For this review, take the finished solid that the model builds, in its own axes (mm). A direction names the side the tool comes from. Round coordinates to 2 decimals unless told otherwise and drop trailing zeros. Write each loop counter-clockwise with the first axis right and the second up, starting at its lowest first coordinate (ties: lowest second). Pieces come first, ordered by that corner, then holes. Notation, with made-up numbers: (-14, 68) -> (25, 68) arc R17 ccw to (25, 93) -> close; hole circle Ø10 at (6.5, -16.5). An arc over 180 degrees is marked (long way). Answer in a Markdown table with one row per item.
from build123d import *

# Parameters (mm, degrees)
SKETCH1_W                             = 69.85
SKETCH1_H                             = 25.4
EXTRUDE1_DEPTH                        = 1.5748
F_1_8_0_125_DIAMETER_HOLE1_AT_2_COUNT = 2
F_1_8_0_125_DIAMETER_HOLE1_AT_2_PITCH = 57.13222
SKETCH4_R                             = 0.635
BOSS_EXTRUDE1_DEPTH                   = 177.8
SKETCH5_W                             = 8.128
SKETCH5_H                             = 8.7376
USB_CONNECTOR_DEPTH                   = 4.1402
SKETCH6_W                             = 10.40639215
SKETCH6_H                             = 6.781860105
CHARGER_DEPTH                         = 20.828
SKETCH7_W                             = 6.585703948
SKETCH7_H                             = 3.257259008
BOSS_EXTRUDE2_DEPTH                   = 10.16
SKETCH8_W                             = 6.5278
SKETCH8_H                             = 15.6718
BOSS_EXTRUDE3_DEPTH                   = 9.8298


with BuildPart() as part:
    # Sketch1 → Extrude1 (new body)
    with BuildSketch(Plane.XY):
        Rectangle(SKETCH1_W, SKETCH1_H)
    extrude(amount=EXTRUDE1_DEPTH)

    # Sketch3 → 1/8 (0.125) Diameter Hole1 (revolve, cut)
    with BuildSketch(Plane(origin=(-25.38222, 9.525, 1.5748), x_dir=(0, -1, 0), z_dir=(1, 0, 0))):
        Polygon((0, 0), (0, 16.955866233), (1.5875, 16.002), (1.5875, 0), align=None)
    f_1_8_0_125_diameter_hole1 = revolve(axis=Axis((-25.38222, 9.525, 7.9248), (0, 0, -1)), mode=Mode.SUBTRACT)

    # 1/8 (0.125) Diameter Hole1 at 2: 1/8 (0.125) Diameter Hole1 ×2
    with Locations(*[(i * F_1_8_0_125_DIAMETER_HOLE1_AT_2_PITCH, 0, 0) for i in range(1, F_1_8_0_125_DIAMETER_HOLE1_AT_2_COUNT)]):
        add(f_1_8_0_125_diameter_hole1, mode=Mode.SUBTRACT)

    # Mirror1: 1/8 (0.125) Diameter Hole1 across plane
    add(f_1_8_0_125_diameter_hole1.mirror(Plane.ZX), mode=Mode.SUBTRACT)

    # Mirror1 copy 1 sketch → Mirror1 copy 1 (revolve, cut)
    with BuildSketch(Plane(origin=(31.75, -9.525, 1.5748), x_dir=(0, 1, 0), z_dir=(1, 0, 0))):
        Polygon((0, 0), (0, -16.955866233), (1.5875, -16.002), (1.5875, 0), align=None)
    revolve(axis=Axis((31.75, -9.525, 7.9248), (0, 0, 1)), mode=Mode.SUBTRACT)

    # Sketch4 → Boss-Extrude1 (add)
    with BuildSketch(Plane(origin=(34.925, 0, 0), x_dir=(0, 0, -1), z_dir=(1, 0, 0))):
        with Locations(Location((-0.772028936, 0, 0), (0, 0, 180))):
            Circle(SKETCH4_R)
    extrude(amount=BOSS_EXTRUDE1_DEPTH)

    # Sketch5 → USB Connector (add)
    with BuildSketch(Plane(origin=(0, 0, 0), x_dir=(-1, 0, 0), z_dir=(0, 0, -1))):
        with Locations((13.072066229, -8.3312)):
            Rectangle(SKETCH5_W, SKETCH5_H)
    extrude(amount=USB_CONNECTOR_DEPTH)

    # Sketch6 → Charger (add)
    with BuildSketch(Plane.XZ.offset(12.7)):
        with Locations((-12.751236003, -1.907476131)):
            Rectangle(SKETCH6_W, SKETCH6_H)
    extrude(amount=CHARGER_DEPTH)

    # Sketch7 → Boss-Extrude2 (add)
    with BuildSketch(Plane.XZ.offset(33.528)):
        with Locations((-12.72298233, -1.628596112)):
            Rectangle(SKETCH7_W, SKETCH7_H)
    extrude(amount=BOSS_EXTRUDE2_DEPTH)

    # Sketch8 → Boss-Extrude3 (add)
    with BuildSketch(Plane.XY.offset(1.5748)):
        with Locations((-31.2801, 0)):
            Rectangle(SKETCH8_W, SKETCH8_H)
    extrude(amount=BOSS_EXTRUDE3_DEPTH)


solid = part.part
1) Consider section B-B on z = 7.5. State the section outline as (x, y) points, then the cut area to 3 significant figures.
Solved:
| item | result |
|---|---|
| outline | (-34.54, -7.84) -> (-28.02, -7.84) -> (-28.02, 7.84) -> (-34.54, 7.84) -> close |
| area | 102 mm² |
2) Consider section C-C on x = 85. State the section outline as (y, z) points (3 decimals), then the cut area to 3 significant figures.
Solved:
| item | result |
|---|---|
| outline | circle Ø1.27 at (0, 0.772) |
| area | 1.27 mm² |
3) For line 1 (Y direction, x = 31.75, z = 0.6); line 2 (X direction, y = 3.5, z = 3.5); line 3 (X direction, y = -22.5, z = -3), list the stretches that pass through material, from the lowest coordinate up. Write a range as [from, to].
Solved:
| item | result |
|---|---|
| line 1 | [-12.7, -11.11], [-7.94, 7.94], [11.11, 12.7] |
| line 2 | [-34.54, -28.02] |
| line 3 | [-17.95, -7.55] |
4) Clearance check with flat-ended pins moving along their axes: pin 1 Ø2 at (y, z) = (-9.5, -1.5) entering from +X; pin 2 Ø1 at (x, y) = (30.5, 2) entering from +Z; pin 3 Ø3 at (y, z) = (-8, 6) entering from +X. State where each tip first meets the part, or that it passes through.
Solved:
| item | result |
|---|---|
| pin 1 | x = -9.01 |
| pin 2 | z = 1.57 |
| pin 3 | x = -28.02 |
5) Consider section A-A on x = 24.5. State the section outline as (y, z) points.
Solved:
| item | result |
|---|---|
| outline | (-12.7, 0) -> (12.7, 0) -> (12.7, 1.57) -> (-12.7, 1.57) -> close |
6) For faces 1 (the flat face through (-7.548, -23, -2)), 2 (the flat face through (-13, -3.962, -2)), 3 (the flat face through (-13, -39, 0)), list the 3-axis set-ups (+Z, -Z, +X, -X, +Y, -Y) from which the entire face can be reached by the end or side of a thin tool; tool diameter is ignored.
Solved:
| item | result |
|---|---|
| face 1 | +Z, -Z, +X, -Y |
| face 2 | -Z, +X, -X, +Y |
| face 3 | +Z, +X, -X, -Y |
